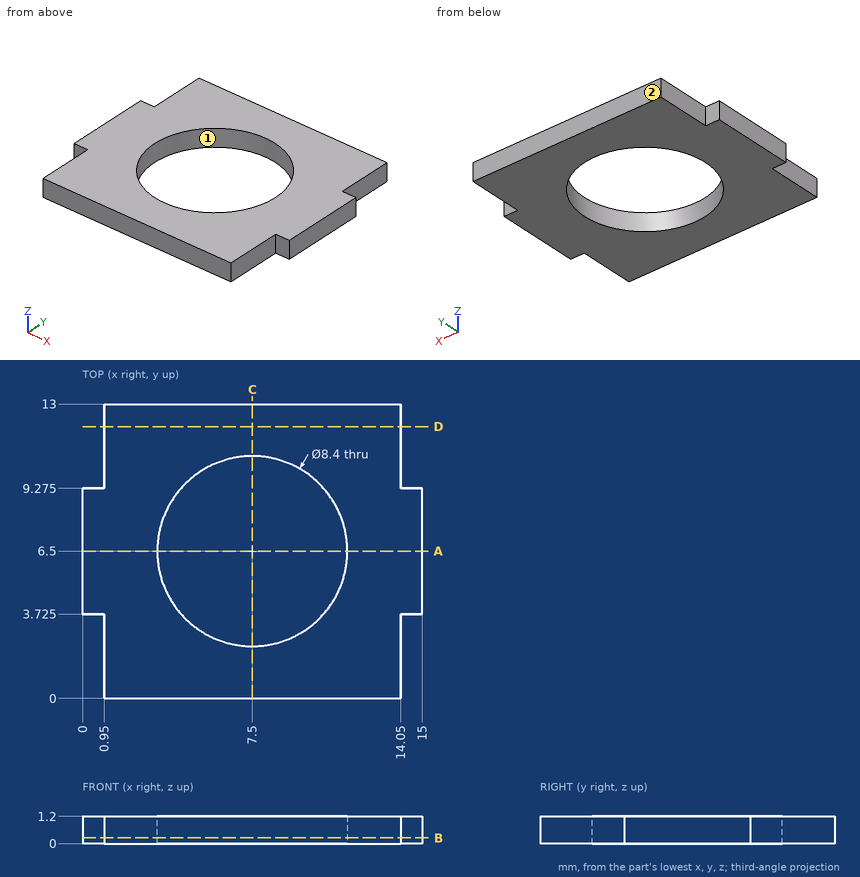
Input: dimensioned drawing with shaded views. Units: mm. Origin: part minimum x, y, z. Round coordinates to 2 decimals unless told otherwise and drop trailing zeros. Order: outer loops, then holes, each group sorted by start corner. A loop starts at its lowest first (then second) coordinate and runs counter-clockwise, first axis right, second up. Notation, with made-up numbers: (7, 30.5) -> (47, 30.5) arc R13 cw to (47, 53.5) -> close; hole circle Ø6 at (-4.5, -19.5). An arc over 180 degrees is marked (long way). One line per item, written item: value. Start each with the question number.
Q1. Pin query (flat end, axial travel): pin 1 (0.6 mm diameter, centred on y = 1.5, z = 1, fed in from -X); pin 2 (0.5 mm diameter, centred on x = 14.5, z = 0.5, fed in from -Y) (3 decimals). Return the tip coordinate at first contact, or that it passes through.
Q2. Section query C-C (x = 7.5). Return the cut outline in (y, z), plus the area to 3 significant figures.
Q3. Section query D-D (y = 12). Return the cut outline in (x, z).
Q4. Draft query along X for the marked faces 1 and 2. Return one class per face: pulls with the +X half, pulls with the -X half, needs draft (parallel to the pull), parting line crosses it, or undercut.
Q5. Section query A-A (y = 6.5). Return the cut outline in (x, z).
Q6. Section query B-B (z = 0.25). Return the cut outline in (x, y) (3 decimals), plus the area to 3 significant figures.
Q7. Material intervals for probe 1 along Y at (x, z) = (7.5, 0.75); probe 2 along X at (y, z) = (2.25, 1.1); probe 3 along Y at (x, z) = (8.75, 0.8), sorted ascending.
Findings below:
1. pin 1: x = 0.95
1. pin 2: y = 3.725
2. outline: (0, 0) -> (2.3, 0) -> (2.3, 1.2) -> (0, 1.2) -> close; (10.7, 0) -> (13, 0) -> (13, 1.2) -> (10.7, 1.2) -> close
2. area: 5.52 mm²
3. outline: (0.95, 0) -> (14.05, 0) -> (14.05, 1.2) -> (0.95, 1.2) -> close
4. face 1: undercut
4. face 2: needs draft
5. outline: (0, 0) -> (3.3, 0) -> (3.3, 1.2) -> (0, 1.2) -> close; (11.7, 0) -> (15, 0) -> (15, 1.2) -> (11.7, 1.2) -> close
6. outline: (0, 3.725) -> (0.95, 3.725) -> (0.95, 0) -> (14.05, 0) -> (14.05, 3.725) -> (15, 3.725) -> (15, 9.275) -> (14.05, 9.275) -> (14.05, 13) -> (0.95, 13) -> (0.95, 9.275) -> (0, 9.275) -> close; hole circle Ø8.4 at (7.5, 6.5)
6. area: 125 mm²
7. probe 1: 0 to 2.3, 10.7 to 13
7. probe 2: 0.95 to 14.05
7. probe 3: 0 to 2.49, 10.51 to 13
